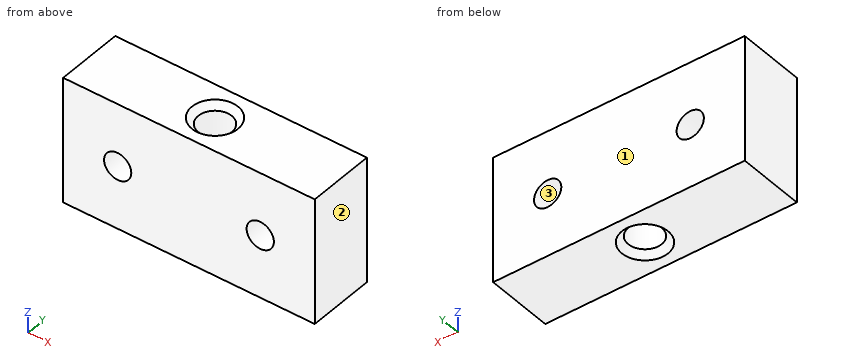
from build123d import *

# Parameters (mm, degrees)
SKETCH1_W           = 60
SKETCH1_H           = 30
SKETCH1_R           = 3.25
BOSS_EXTRUDE1_DEPTH = 16
SKETCH2_R           = 4
CUT_EXTRUDE1_DEPTH  = 31
CHAMFER1_SIZE       = 1.5


with BuildPart() as part:
    # Sketch1 → Boss-Extrude1 (new body)
    with BuildSketch(Plane(origin=(0, 0, 0), x_dir=(1, 0, 0), z_dir=(0, 1, 0))):
        with Locations((30, 15)):
            Rectangle(SKETCH1_W, SKETCH1_H)
        with Locations((13, 15)):
            Circle(SKETCH1_R, mode=Mode.SUBTRACT)
        with Locations((47, 15)):
            Circle(SKETCH1_R, mode=Mode.SUBTRACT)
    extrude(amount=BOSS_EXTRUDE1_DEPTH)

    # Sketch2 → Cut-Extrude1 (cut, through all)
    with BuildSketch(Plane.XY):
        with Locations((30, 8)):
            Circle(SKETCH2_R)
    extrude(amount=-CUT_EXTRUDE1_DEPTH, mode=Mode.SUBTRACT)

    # Chamfer1
    chamfer1_edges = [part.edges().sort_by_distance(p)[0] for p in [
        (26, 8, -30),
        (26, 8, 0),
    ]]
    chamfer(chamfer1_edges, length=CHAMFER1_SIZE)


solid = part.part
Verification items for the finished model (mm, model axes). Face numbers are marked on the shaded views. Give positions to 0.01 mm unless a question says otherwise; leave off trailing zeros. Write each loop counter-clockwise with the first axis right and the second up, starting at its lowest first coordinate (ties: lowest second). Pieces come first, ordered by that corner, then holes.
(1) Mould release check, pull along X, two halves, no side actions. Record for the marked faces 1, 2 and 3: +X half, -X half, draft (parallel to the pull), parting line (faces both ways), or undercut.
(2) Material ranges on line 1 (X direction, y = 10.75, z = -15); line 2 (X direction, y = 1.25, z = -16); line 3 (X direction, y = 7.25, z = -15), recorded low to high.
(3) Gauge pin test, flat ends, axial feed: pin 1 (8.5 mm diameter, centred on x = 47, z = -15, fed in from +Y); pin 2 (9 mm diameter, centred on x = 30, y = 8, fed in from +Z). Record the tip position at first contact, or that the pin passes through.
(4) Cross-section at D-D (y = 14.25). Enter the section's corners in (x, z), plus the area to 3 significant figures.
(5) Cross-section at A-A (z = -15). Enter the section's corners in (x, y).
(6) Cross-section at B-B (x = 47). Enter the section's corners in (y, z), plus the area to 3 significant figures.
(7) Cross-section at C-C (y = 8). Enter the section's corners in (x, z).
Worked out:
1. face 1: draft
1. face 2: +X half
1. face 3: undercut
2. line 1: x = 0 to 9.75, 16.25 to 27.1, 32.9 to 43.75, 50.25 to 60
2. line 2: x = 0 to 9.91, 16.09 to 43.91, 50.09 to 60
2. line 3: x = 0 to 9.75, 16.25 to 26.07, 33.93 to 43.75, 50.25 to 60
3. pin 1: stops at y = 16
3. pin 2: stops at z = -1
4. outline: (0, -30) - (60, -30) - (60, 0) - (0, 0) - close; hole circle Ø6.5 at (13, -15); hole circle Ø6.5 at (47, -15)
4. area: 1,730 mm2
5. outline: (0, 0) - (9.75, 0) - (9.75, 16) - (0, 16) - close; (16.25, 0) - (43.75, 0) - (43.75, 16) - (16.25, 16) - close; (50.25, 0) - (60, 0) - (60, 16) - (50.25, 16) - close; hole circle Ø8 at (30, 8)
6. outline: (0, -30) - (16, -30) - (16, -18.25) - (0, -18.25) - close; (0, -11.75) - (16, -11.75) - (16, 0) - (0, 0) - close
6. area: 376 mm2
7. outline: (0, -30) - (24.5, -30) - (26, -28.5) - (26, -1.5) - (24.5, 0) - (0, 0) - close; (34, -28.5) - (35.5, -30) - (60, -30) - (60, 0) - (35.5, 0) - (34, -1.5) - close; hole circle Ø6.5 at (13, -15); hole circle Ø6.5 at (47, -15)
